The listing builds one solid part. Answer for the finished solid, in the listing's coordinates (mm). A direction names the side the tool comes from. Coordinates: 2 decimals unless noted, no trailing zeros. Order: outer loops, then holes, each group sorted by start corner. A loop starts at its lowest first (then second) coordinate and runs counter-clockwise, first axis right, second up. Notation, with made-up numbers: (-35, 44) -> (-10, 44) arc R34 cw to (-10, 75) -> close; hole circle Ø10 at (69.25, -30). An arc over 180 degrees is marked (long way). Answer in a Markdown table with one row per item. Add a question column.
```python
from build123d import *

# Parameters (mm, degrees)
CROQUIS1_W              = 985
CROQUIS1_H              = 135
SALIENTE_EXTRUIR1_DEPTH = 12
CORTAR_EXTRUIR1_DEPTH   = 47.5
CROQUIS3_R              = 65
CORTAR_EXTRUIR2_DEPTH   = 29


with BuildPart() as part:
    # Croquis1 → Saliente-Extruir1 (new body)
    with BuildSketch(Plane.XY):
        with Locations((-492.5, 67.5)):
            Rectangle(CROQUIS1_W, CROQUIS1_H)
    extrude(amount=SALIENTE_EXTRUIR1_DEPTH)

    # Croquis2 → Cortar-Extruir1 (cut)
    with BuildSketch(Plane(origin=(0, 135, 0), x_dir=(1, 0, 0), z_dir=(0, 1, 0))):
        with BuildLine():
            Line((-25.534833896, 0), (-108.465166104, 0))
            ThreePointArc((-108.465166104, 0), (-103.062225626, -6.494730354), (-96.654004789, -12))
            Line((-96.654004789, -12), (-37.345995211, -12))
            ThreePointArc((-37.345995211, -12), (-30.937774374, -6.494730354), (-25.534833896, 0))
        make_face()
    extrude(amount=-CORTAR_EXTRUIR1_DEPTH, mode=Mode.SUBTRACT)

    # Croquis3 → Cortar-Extruir2 (cut)
    with BuildSketch(Plane(origin=(0, 82, 0), x_dir=(1, 0, 0), z_dir=(0, 1, 0))):
        with Locations((-67, -58)):
            Circle(CROQUIS3_R)
    extrude(amount=-CORTAR_EXTRUIR2_DEPTH, mode=Mode.SUBTRACT)


solid = part.part
```
Q1. Straight lines are drawn through the part: line 1 (Y direction, x = -107, z = 11.25); line 2 (X direction, y = 57, z = 4); line 3 (X direction, y = 113.5, z = 9). For each, find the intervals that lie inside material, in ascending order.
Q2. Determine the mould class of faces 3 (the face through (-28.77, 67.7, 5.43)), 4 (the face through (-499, 68, 12)) for opening direction Y: +Y half, -Y half, draft (parallel to the pull), parting line (faces both ways), or undercut.
Q3. A cutting plane is placed at B-B (z = 7.25). Determine the outline of the cut face in (x, y).
Q4. A cutting plane is placed at C-C (y = 121). Determine the outline of the cut face in (x, z).
Q5. Given pin 1 (3.5 mm diameter, centred on x = -56.5, z = 7.5, fed in from +Y), flat-ended and moving along its own axis, determine where the tip first touches the part or whether it passes through.
Q6. For faces 1 (the face through (-104.99, 67.7, 5.26)), 2 (the face through (-499, 68, 0)), determine the directions among +Z, -Z, +X, -X, +Y, -Y from which every point of the face is accessible in a straight line to the end or side of a thin tool.
Q7. A cutting plane is placed at A-A (y = 64). Determine the outline of the cut face in (x, z), then the cut area to 3 significant figures.
Returned:
| question | item | result |
|---|---|---|
| 1 | line 1 | y = 0 to 53, 82 to 135 |
| 1 | line 2 | x = -985 to -103.18, -30.82 to 0 |
| 1 | line 3 | x = -985 to -100.41, -33.59 to 0 |
| 2 | face 3 | undercut |
| 2 | face 4 | draft |
| 3 | outline | (-985, 0) -> (0, 0) -> (0, 135) -> (-31.7, 135) -> (-31.7, 87.5) -> (-102.3, 87.5) -> (-102.3, 135) -> (-985, 135) -> close; hole (-107.61, 53) -> (-26.39, 53) -> (-26.39, 82) -> (-107.61, 82) -> close |
| 4 | outline | (-985, 0) -> (-108.47, 0) arc R50.6 cw to (-96.65, 12) -> (-985, 12) -> close; (-37.35, 12) arc R50.6 cw to (-25.53, 0) -> (0, 0) -> (0, 12) -> close |
| 5 | pin 1 | stops at y = 87.5 |
| 6 | face 1 | +Z |
| 6 | face 2 | -Z, +X, -X, +Y, -Y |
| 7 | outline | (-985, 0) -> (-96.34, 0) arc R65 cw to (-112.92, 12) -> (-985, 12) -> close; (-37.66, 0) -> (0, 0) -> (0, 12) -> (-21.08, 12) arc R65 cw to start |
| 7 | area | 10,900 mm² |
